The listing builds one solid part. Answer for the finished solid, in the listing's coordinates (mm). A direction names the side the tool comes from. Round coordinates to 2 decimals unless told otherwise and drop trailing zeros. Loops run counter-clockwise (first coordinate to the right, second up) from the corner with the lowest first, then second, coordinate; pieces in that order, holes last. Notation, with made-up numbers: (-16.5, 1) -> (16.5, 1) arc R24 ccw to (16.5, 15) -> close; hole circle Ø7 at (25, -23.75). An arc over 180 degrees is marked (long way). Use a Markdown table: item, result. Add a question column.
Q1. Section C-C on y = 11 is taken. Give the vertices of the cut face in (x, z), then the cut area to 3 significant figures.
Q2. For a pull along Z with two mould halves and no side action, classify faces 3 (the flat face through (12, 8, 34)), 4 (the cylindrical face through (12.325, 5.044, 17.661)), 5 (the cylindrical face through (12.325, 5.867, 0.511)), 6 (the flat face through (12, 15, 28)) as released by +Z, released by -Z, zero draft, split by the parting line, or undercut.
Q3. Given pin 1 Ø4 at (x, y) = (19.5, 11) entering from -Z; pin 2 Ø5 at (y, z) = (9, 9) entering from -X; pin 3 Ø7 at (x, z) = (6.25, 28) entering from -Y; pin 4 Ø4 at (x, y) = (15, 13) entering from -Z, each flat-ended and moving along its own axis, determine where each tip first touches the part or whether it passes through.
Q4. Section B-B on x = 18.75 is taken. Give the vertices of the cut face in (y, z).
Q5. Section A-A on z = 28 is taken. Give the vertices of the cut face in (x, y).
Q6. Consider line 1 (Z direction, x = 18.75, y = 10.25); line 2 (Z direction, x = 6.25, y = 2.25); line 3 (Z direction, x = 6.25, y = 6.25). Determine where each line is inside the solid, lowest interval first.
Q7. Which of the six approach directions +Z, -Z, +X, -X, +Y, -Y give full straight-line access (tool end or side, diameter ignored) to faces 1 (the cylindrical face through (7.288, 7.395, 26.004)), 2 (the flat face through (12, 12, 22))?
Q8. Section D-D on x = 9 is taken. Give the vertices of the cut face in (y, z), then the cut area to 3 significant figures.
from build123d import *

# Parameters (mm, degrees)
F1_DEPTH = 25
F2_R     = 2.25
F3_DEPTH = 28.7
F4_R     = 4.25
F4_R_2   = 2.25
F4_W     = 25
F4_H     = 32
F5_DEPTH = 2


with BuildPart() as f1:
    # F0 (on Right) → F1 (new body)
    with BuildSketch(Plane.YZ):
        with BuildLine():
            ThreePointArc((0, 2), (0.585786, 0.585786), (2, 0))
            Line((2, 0), (2.3, 0))
            ThreePointArc((2.3, 0), (5.916074, 0.525682), (9.232793, 2.059211))
            ThreePointArc((9.232793, 2.059211), (5.014177, 6.623749), (8.5, 11.769696))
            Line((8.5, 11.769696), (8.5, 12.230304))
            ThreePointArc((8.5, 12.230304), (5.057911, 17.758788), (10, 22))
            Line((10, 22), (15, 22))
            Line((15, 22), (15, 34))
            Line((15, 34), (0, 34))
            Line((0, 34), (0, 2))
        make_face()
    extrude(amount=F1_DEPTH)

    # F2 (on face) → F3 (cut)
    with BuildSketch(Plane.XZ):
        with Locations((6.25, 28)):
            Circle(F2_R)
        with Locations((18.75, 28)):
            Circle(F2_R)
    extrude(amount=-F3_DEPTH, mode=Mode.SUBTRACT)

    # F4 (on face) → F5 (join)
    with BuildSketch(Plane.XZ):
        with Locations((6.25, 28)):
            Circle(F4_R)
        with Locations((6.25, 28)):
            Circle(F4_R_2, mode=Mode.SUBTRACT)
        with Locations((12.5, 18)):
            Rectangle(F4_W, F4_H)
        with Locations((6.25, 28)):
            Circle(F4_R, mode=Mode.SUBTRACT)
        with Locations((18.75, 28)):
            Circle(F4_R, mode=Mode.SUBTRACT)
    extrude(amount=-F5_DEPTH)


solid = f1.part
Checked values:
| question | item | result |
|---|---|---|
| 1 | outline | (0, 22) -> (25, 22) -> (25, 34) -> (0, 34) -> close; hole circle Ø4.5 at (6.25, 28); hole circle Ø4.5 at (18.75, 28) |
| 1 | area | 268 mm2 |
| 2 | face 3 | released by +Z |
| 2 | face 4 | undercut |
| 2 | face 5 | released by -Z |
| 2 | face 6 | zero draft |
| 3 | pin 1 | stops at z = 1.91 |
| 3 | pin 2 | passes through |
| 3 | pin 3 | stops at y = 0 |
| 3 | pin 4 | stops at z = 22 |
| 4 | outline | (0, 2) arc R2 ccw to (2, 0) -> (2.3, 0) arc R12.7 ccw to (9.23, 2.06) arc R5 cw to (8.5, 11.77) -> (8.5, 12.23) arc R5 cw to (10, 22) -> (15, 22) -> (15, 25.75) -> (0, 25.75) -> close; (0, 30.25) -> (15, 30.25) -> (15, 34) -> (0, 34) -> close |
| 5 | outline | (0, 0) -> (4, 0) -> (4, 15) -> (0, 15) -> close; (8.5, 0) -> (16.5, 0) -> (16.5, 15) -> (8.5, 15) -> close; (21, 0) -> (25, 0) -> (25, 15) -> (21, 15) -> close |
| 6 | line 1 | z = 22 to 25.75, 30.25 to 34 |
| 6 | line 2 | z = 0 to 25.75, 30.25 to 34 |
| 6 | line 3 | z = 0.63 to 3.69, 10.31 to 13.69, 20.31 to 25.75, 30.25 to 34 |
| 7 | face 1 | +Y, -Y |
| 7 | face 2 | -Z, +X, -X, +Y |
| 8 | outline | (0, 2) arc R2 ccw to (2, 0) -> (2.3, 0) arc R12.7 ccw to (9.23, 2.06) arc R5 cw to (8.5, 11.77) -> (8.5, 12.23) arc R5 cw to (10, 22) -> (15, 22) -> (15, 34) -> (0, 34) -> close |
| 8 | area | 314 mm2 |
